Source: CAD feature listing. Evaluate the final solid. Frame: model axes, mm. A direction names the side the tool comes from. Give positions to 0.01 mm unless a question says otherwise; leave off trailing zeros. Order: outer loops, then holes, each group sorted by start corner. A loop starts at its lowest first (then second) coordinate and runs counter-clockwise, first axis right, second up.
from build123d import *

# Parameters (mm, degrees)
BOSS_EXTRUDE1_DEPTH             = 10
SKETCH2_R                       = 5
CUT_EXTRUDE1_DEPTH              = 11
FILLET1_R                       = 3
CUT_EXTRUDE4_DEPTH              = 11
CUT_EXTRUDE5_DEPTH              = 8
FILLET2_R                       = 3
F_3_0MM_DOWEL_HOLE1_AT_2_COUNT  = 2
F_3_0MM_DOWEL_HOLE1_AT_2_PITCH  = 40
TAP_DRILL_FOR_M3X0_5_TAP1_D     = 2.5
TAP_DRILL_FOR_M3X0_5_TAP1_DEPTH = 2
F_3_0MM_DOWEL_HOLE3_D           = 3
F_3_0MM_DOWEL_HOLE4_D           = 3
F_3_0MM_DOWEL_HOLE4_DEPTH       = 2


with BuildPart() as part:
    # Sketch1 → Boss-Extrude1 (new body)
    with BuildSketch(Plane(origin=(0, 0, 0), x_dir=(1, 0, 0), z_dir=(0, 1, 0))):
        Polygon((0, 88), (0, 8), (8, 0), (88, 0), (96, 8), (96, 88), (88, 96), (8, 96), align=None)
    extrude(amount=BOSS_EXTRUDE1_DEPTH)

    # Sketch2 → Cut-Extrude1 (cut, through all)
    with BuildSketch(Plane(origin=(0, 0, 0), x_dir=(-1, 0, 0), z_dir=(0, -1, 0))):
        with BuildLine():
            Line((-45.411809549, 57.659258263), (-19.071067812, 84))
            Line((-19.071067812, 84), (-76.928932188, 84))
            Line((-76.928932188, 84), (-50.588190451, 57.659258263))
            ThreePointArc((-50.588190451, 57.659258263), (-48, 58), (-45.411809549, 57.659258263))
        make_face()
        with BuildLine():
            Line((-12, 76.928932188), (-38.340741737, 50.588190451))
            ThreePointArc((-38.340741737, 50.588190451), (-38.085551386, 49.305261922), (-38, 48))
            ThreePointArc((-38, 48), (-38.085551386, 46.694738078), (-38.340741737, 45.411809549))
            Line((-38.340741737, 45.411809549), (-12, 19.071067812))
            Line((-12, 19.071067812), (-12, 76.928932188))
        make_face()
        with BuildLine():
            Line((-19.071067812, 12), (-45.411809549, 38.340741737))
            ThreePointArc((-45.411809549, 38.340741737), (-48, 38), (-50.588190451, 38.340741737))
            Line((-50.588190451, 38.340741737), (-76.928932188, 12))
            Line((-76.928932188, 12), (-19.071067812, 12))
        make_face()
        with BuildLine():
            ThreePointArc((-57.659258263, 45.411809549), (-58, 48), (-57.659258263, 50.588190451))
            Line((-57.659258263, 50.588190451), (-84, 76.928932188))
            Line((-84, 76.928932188), (-84, 19.071067812))
            Line((-84, 19.071067812), (-57.659258263, 45.411809549))
        make_face()
        with Locations((-48, 48)):
            Circle(SKETCH2_R)
    extrude(amount=-CUT_EXTRUDE1_DEPTH, mode=Mode.SUBTRACT)

    # Fillet1
    fillet1_edges = [part.edges().sort_by_distance(p)[0] for p in [
        (50.588190451, 5, -38.340741737),
        (45.411809549, 5, -38.340741737),
        (19.071067812, 5, -12),
        (76.928932188, 5, -12),
        (38.340741737, 5, -45.411809549),
        (38.340741737, 5, -50.588190451),
        (12, 5, -76.928932188),
        (12, 5, -19.071067812),
        (57.659258263, 5, -50.588190451),
        (57.659258263, 5, -45.411809549),
        (84, 5, -19.071067812),
        (84, 5, -76.928932188),
        (45.411809549, 5, -57.659258263),
        (50.588190451, 5, -57.659258263),
        (76.928932188, 5, -84),
        (19.071067812, 5, -84),
    ]]
    fillet(fillet1_edges, radius=FILLET1_R)

    # Sketch5 → Cut-Extrude4 (cut, through all)
    with BuildSketch(Plane(origin=(0, 10, 0), x_dir=(1, 0, 0), z_dir=(0, 1, 0))):
        Polygon((8, 0), (8, 20.5), (0, 20.5), (0, 8), align=None)
        Polygon((96, 8), (88, 0), (88, 20.5), (96, 20.5), align=None)
        Polygon((96, 75.5), (88, 75.5), (88, 96), (96, 88), align=None)
        Polygon((8, 96), (8, 75.5), (0, 75.5), (0, 88), align=None)
    extrude(amount=-CUT_EXTRUDE4_DEPTH, mode=Mode.SUBTRACT)

    # Sketch6 → Cut-Extrude5 (cut)
    with BuildSketch(Plane(origin=(0, 10, 0), x_dir=(1, 0, 0), z_dir=(0, 1, 0))):
        Polygon((86, 73.5), (86, 94), (10, 94), (10, 73.5), (2, 73.5), (2, 22.5), (10, 22.5), (10, 2), (86, 2), (86, 22.5), (94, 22.5), (94, 73.5), align=None)
    extrude(amount=-CUT_EXTRUDE5_DEPTH, mode=Mode.SUBTRACT)

    # Fillet2
    fillet2_edges = [part.edges().sort_by_distance(p)[0] for p in [
        (8, 5, -75.5),
        (88, 5, -75.5),
        (88, 5, -20.5),
        (8, 5, -20.5),
        (94, 6, -73.5),
        (94, 6, -22.5),
        (86, 6, -2),
        (10, 6, -2),
        (2, 6, -22.5),
        (2, 6, -73.5),
        (10, 6, -94),
        (86, 6, -94),
    ]]
    fillet(fillet2_edges, radius=FILLET2_R)

    # Sketch13 → Ø3.0mm Dowel Hole1 (revolve, cut)
    with BuildSketch(Plane(origin=(28, 6, 0), x_dir=(0, -1, 0), z_dir=(1, 0, 0))):
        Polygon((0, 0), (0, 8.401290929), (1.5, 7.5), (1.5, 0), align=None)
    f_3_0mm_dowel_hole1 = revolve(axis=Axis((28, 6, 6.35), (0, 0, -1)), mode=Mode.SUBTRACT)

    # Ø3.0mm Dowel Hole1 at 2: Ø3.0mm Dowel Hole1 ×2
    with Locations(*[(i * F_3_0MM_DOWEL_HOLE1_AT_2_PITCH, 0, 0) for i in range(1, F_3_0MM_DOWEL_HOLE1_AT_2_COUNT)]):
        add(f_3_0mm_dowel_hole1, mode=Mode.SUBTRACT)

    # Tap Drill for M3x0.5 Tap1
    with Locations(Plane.ZY):
        with Locations((-68, 6), (-28, 6)):
            Hole(TAP_DRILL_FOR_M3X0_5_TAP1_D / 2, depth=TAP_DRILL_FOR_M3X0_5_TAP1_DEPTH)

    # Mirror1: Ø3.0mm Dowel Hole1 across plane
    add(f_3_0mm_dowel_hole1.mirror(Plane.XY.offset(-48)), mode=Mode.SUBTRACT)

    # Mirror1 copy 1 sketch → Mirror1 copy 1 (revolve, cut)
    with BuildSketch(Plane(origin=(68, 6, -96), x_dir=(0, -1, 0), z_dir=(1, 0, 0))):
        Polygon((0, 0), (0, -8.401290929), (1.5, -7.5), (1.5, 0), align=None)
    revolve(axis=Axis((68, 6, -102.35), (0, 0, -1)), mode=Mode.SUBTRACT)

    # Ø3.0mm Dowel Hole3 (through all)
    with Locations(Plane(origin=(78, 0, -18), x_dir=(0, 0, -1), z_dir=(0, -1, 0))):
        with Locations((0, 0), (60, 0), (60, -60), (0, -60)):
            Hole(F_3_0MM_DOWEL_HOLE3_D / 2)

    # Ø3.0mm Dowel Hole4
    with Locations(Plane(origin=(96, 6, -68), x_dir=(0, 0, 1), z_dir=(1, 0, 0))):
        with Locations((0, 0), (40, 0)):
            Hole(F_3_0MM_DOWEL_HOLE4_D / 2, depth=F_3_0MM_DOWEL_HOLE4_DEPTH)


solid = part.part
1) Pull-direction query (X, two-part tool) for faces 1 (the face through (3, 5, -75.5)), 2 (the face through (7, 6, -22.5)), 3 (the face through (7.14, 4.93, -19.6)); classes: +X half, -X half, draft (parallel to the pull), parting line (faces both ways), or undercut.
Checks:
face 1: draft
face 2: undercut
face 3: -X half
2) Section query A-A on x = 63. Output: boundary loops of the cut face in (y, z), and give its area (3 significant figures).
Checks:
outline: (0, -96) - (10, -96) - (10, -94) - (2, -94) - (2, -84) - (0, -84) - close; (0, -70.07) - (2, -70.07) - (2, -55.93) - (0, -55.93) - close; (0, -40.07) - (2, -40.07) - (2, -25.93) - (0, -25.93) - close; (0, -12) - (2, -12) - (2, -2) - (10, -2) - (10, 0) - (0, 0) - close
area: 137 mm2
3) Ray query, L1, parallel to X at y = 6, z = -0.35; L2, parallel to X at y = 2.5, z = -11; L3, parallel to X at y = 7.25, z = -34.5. Return the intervals inside material, ascending.
Checks:
L1: x = 8 to 26.5, 29.5 to 66.5, 69.5 to 88
L2: x = 8 to 10, 86 to 88
L3: x = 0 to 2, 94 to 96
4) Reachability of faces 4 (the face through (88, 5, -87)), 5 (the face through (86, 6, -14)), 6 (the face through (94.99, 5.55, -69.43)), 7 (the face through (72.476, 1.014, -82.102)), 8 (the face through (8, 5, -87)) from +Z, -Z, +X, -X, +Y, -Y: full face, straight path, thin tool, end or side. Return the list, or none.
Checks:
face 4: -Z, +X, +Y, -Y
face 5: +Y
face 6: +X
face 7: +Y, -Y
face 8: -Z, -X, +Y, -Y
5) Section query D-D on y = 6. State how many separate pieces and enclosed holes the cut face has, and give its area (3 significant figures).
Checks:
separate pieces: 8
enclosed holes: 0
area: 729 mm2
6) Section query C-C on x = 28. Output: boundary loops of the cut face in (y, z).
Checks:
outline: (0, -96) - (4.5, -96) - (4.5, -94) - (2, -94) - (2, -84) - (0, -84) - close; (0, -75.07) - (2, -75.07) - (2, -60.93) - (0, -60.93) - close; (0, -35.07) - (2, -35.07) - (2, -20.93) - (0, -20.93) - close; (0, -12) - (2, -12) - (2, -2) - (4.5, -2) - (4.5, 0) - (0, 0) - close; (7.5, -96) - (10, -96) - (10, -94) - (7.5, -94) - close; (7.5, -2) - (10, -2) - (10, 0) - (7.5, 0) - close
7) Section query B-B on z = -82. Output: boundary loops of the cut face in (x, y).
Checks:
outline: (8, 0) - (23.49, 0) - (23.49, 2) - (10, 2) - (10, 10) - (8, 10) - close; (72.51, 0) - (88, 0) - (88, 10) - (86, 10) - (86, 2) - (72.51, 2) - close
8) First-contact query: pin 1 Ø8 at (x, z) = (84.5, -49) entering from +Y; pin 2 Ø5.5 at (x, y) = (3.5, 3) entering from +Z; pin 3 Ø2.5 at (x, z) = (18, -18) entering from -Y; pin 4 Ø5.5 at (x, y) = (93.5, 5.5) entering from +Z. Flat tips, straight axial feed; report the tip coordinate or a pass-through.
Checks:
pin 1: stops at y = 2
pin 2: stops at z = -20.23
pin 3: passes through
pin 4: stops at z = -20.49
